Design review of the part shown in the three views and the two pictorial views. Dimensions are in mm from the part's minimum x, y and z. Round coordinates to 2 decimals unless told otherwise and drop trailing zeros. Order: outer loops, then holes, each group sorted by start corner. A loop starts at its lowest first (then second) coordinate and runs counter-clockwise, first axis right, second up. Notation, with made-up numbers: M 81,-17 L 134,-17 A16 cw 134,9 Z; hole C 14,63.25 d9. An arc over 180 degrees is marked long. Use a Markdown table: item, result. Add a question column.
(1) For pin 1 (6 mm diameter, centred on y = 339, z = 113, fed in from +X), flat-tipped, find the tip position at first contact; note if it passes through.
(2) Take a section at B-B (z = 409). Write out the cut boundary in (x, y).
(3) To check wall thickness, follow probe 1 along X at (y, z) = (195.5, 325.5). State the ranges of the line that lie inside material, in increasing order. Write a range as from..to.
(4) Take a section at A-A (y = 292). Write out the cut boundary in (x, z), then the cut area to 3 significant figures.
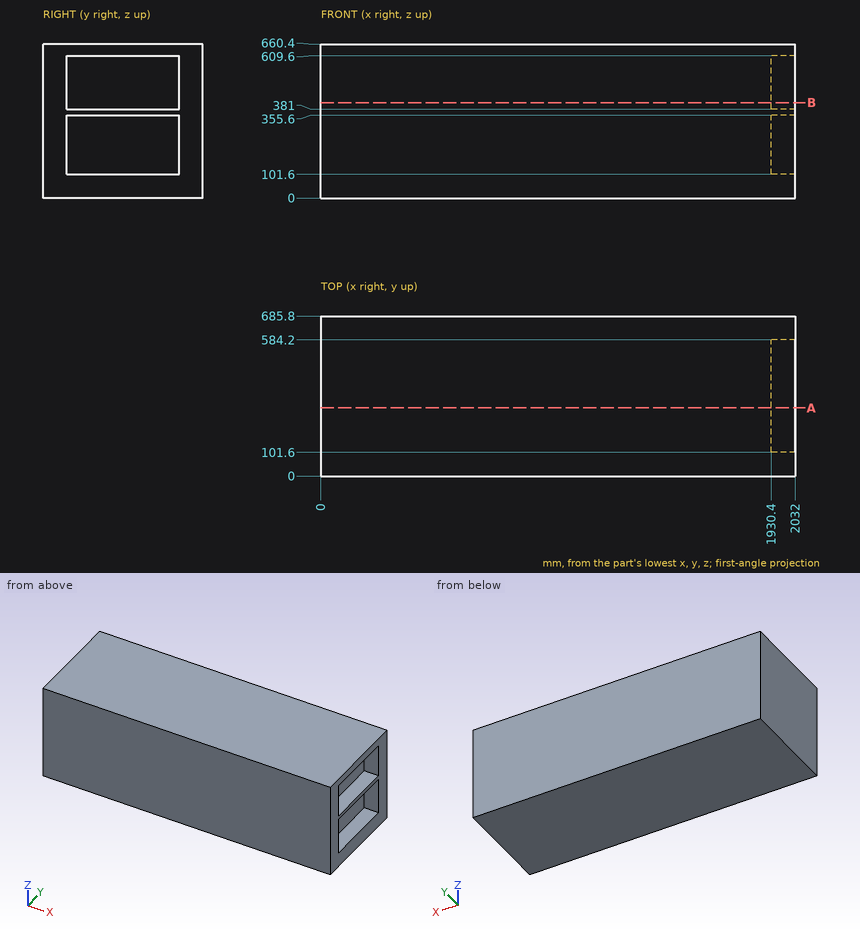
Verdict:
| question | item | result |
|---|---|---|
| 1 | pin 1 | stops at x = 1930.4 |
| 2 | outline | M 0,0 L 2032,0 L 2032,101.6 L 1930.4,101.6 L 1930.4,584.2 L 2032,584.2 L 2032,685.8 L 0,685.8 Z |
| 3 | probe 1 | x = 0..1930.4 |
| 4 | outline | M 0,0 L 2032,0 L 2032,101.6 L 1930.4,101.6 L 1930.4,355.6 L 2032,355.6 L 2032,381 L 1930.4,381 L 1930.4,609.6 L 2032,609.6 L 2032,660.4 L 0,660.4 Z |
| 4 | area | 1,290,000 mm^2 |
